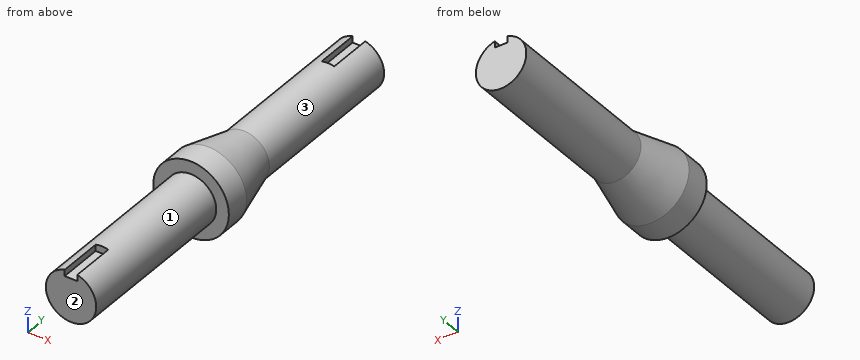
from build123d import *

# Parameters (mm, degrees)
F0_R     = 4
F1_DEPTH = 65
F3_R     = 6
F4_DEPTH = 4
F5_SIZE2 = 1.99999
F5_SIZE  = 7.99999
F7_DEPTH = 7


# Not quite as in the source:
# - a fillet or chamfer is up to 0.001 mm smaller than in the source, because OpenCascade refuses the exact size
# - a pattern or mirror of a feature is missing from the dataset's text; its kind, count and spacing are read off the source's solid


with BuildPart() as f1:
    # F0 (on Front) → F1 (new body)
    with BuildSketch(Plane.XZ):
        Circle(F0_R)
    extrude(amount=F1_DEPTH)

    # F3 (on offset) → F4 (join)
    with BuildSketch(Plane.XZ.offset(37.9)):
        Circle(F3_R)
    extrude(amount=-F4_DEPTH)

    # F5 (size 8 and 2 in the source; OpenCascade refuses exactly that, so slightly less here)
    f5_edges = [f1.edges().sort_by_distance(p)[0] for p in [
        (-4, -33.9, 0),
    ]]
    f5_side = f1.faces().sort_by_distance((-4, -16.95, 0))[0]
    chamfer(f5_edges, length=F5_SIZE, length2=F5_SIZE2, reference=f5_side)

    # F6 (on face) → F7 (cut)
    with BuildSketch(Plane.XZ.offset(65)):
        Polygon((0, 4.4108442962), (-1, 3.8729833462), (-1, 2.8729833462), (1, 2.8729833462), (1, 3.8729833462), align=None)
    f7 = extrude(amount=-F7_DEPTH, mode=Mode.SUBTRACT)

    # F7_copies: F7 across plane
    add(f7.mirror(Plane.ZX.offset(-32.5)), mode=Mode.SUBTRACT)


solid = f1.part
Part model, mm, in its own coordinate system. Face numbers are marked on the shaded views. A direction names the side the tool comes from. Coordinates: 2 decimals unless noted, no trailing zeros. Write each loop counter-clockwise with the first axis right and the second up, starting at its lowest first coordinate (ties: lowest second). Pieces come first, ordered by that corner, then holes. Notation, with made-up numbers: (29.25, 29) - (70.25, 29) arc R12 cw to (70.25, 33) - close; hole circle Ø1 at (-11.5, 32.25). An arc over 180 degrees is marked (long way). Put each result on its own line as item: value.
1. Probe line 1 along X through (y, z) = (-53, 0); line 2 along X through (y, z) = (-31, -2); line 3 along Z through (x, y) = (3, -44). List the from-to ranges inside material, lowest first. Write a range as [from, to].
Final values:
line 1: x = [-4, 4]
line 2: x = [-4.88, 4.88]
line 3: z = [-2.65, 2.65]
2. Flat gauge pins, fed straight in: pin 1 Ø0.6 at (x, y) = (0, -60.5) entering from +Z; pin 2 Ø5 at (y, z) = (-14, -4) entering from -X; pin 3 Ø1.1 at (y, z) = (-60, 3.5) entering from -X. Where does each tip first touch, or does it go through?
Final values:
pin 1: stops at z = 2.87
pin 2: stops at x = -3.71
pin 3: stops at x = -2.7
3. 3-axis set-ups, long thin cutter, end or side, ignore diameter. For the marked faces 1, 2 and 3: which of +Z, -Z, +X, -X, +Y, -Y reach the whole face in a straight line?
Final values:
face 1: -Y
face 2: +Z, -Z, +X, -X, -Y
face 3: +Y
4. Band-saw the part on C-C (y = -18). Write the cut outline in (x, z).
Final values:
outline: circle Ø8 at (0, 0)
